Geometry: see drawing. Coordinates: mm, zero at the bounding-box minimum. A direction names the side the tool comes from. Round coordinates to 2 decimals unless told otherwise and drop trailing zeros. Order: outer loops, then holes, each group sorted by start corner. A loop starts at its lowest first (then second) coordinate and runs counter-clockwise, first axis right, second up. Notation, with made-up numbers: (39, -17) -> (80, -17) arc R20 cw to (80, -12) -> close; hole circle Ø2 at (19, -10). An arc over 180 degrees is marked (long way). One line per item, written item: value. Start each with the question number.
1) Section C-C (z = 28). Return the cut outline in (x, y) (1 decimal).
2) Section A-A (x = 4.25). Return the cut outline in (y, z), and give its area (3 significant figures).
3) Section B-B (y = 3.5). Return the cut outline in (x, z).
4) Pin query (flat end, axial travel): P1, Ø1, axis at y = 3.5, z = 32.5, coming from the +X side; P2, Ø1, axis at x = 3.5, z = 47.5, coming from the -Y side. Return the tip coordinate at first contact, or that it passes through.
5) Reachability of the marked faces 1, 2 and 3 from +Z, -Z, +X, -X, +Y, -Y: full face, straight path, thin tool, end or side. Return the list, or none.
6) Ray query, L1, parallel to Z at x = 10, y = 8.25; L2, parallel to Y at x = 5.75, z = 11.5; L3, parallel to Y at x = 6.5, z = 53 (1 decimal). Return the intervals inside material, ascending.
7) Section D-D (z = 68.5). Return the cut outline in (x, y).
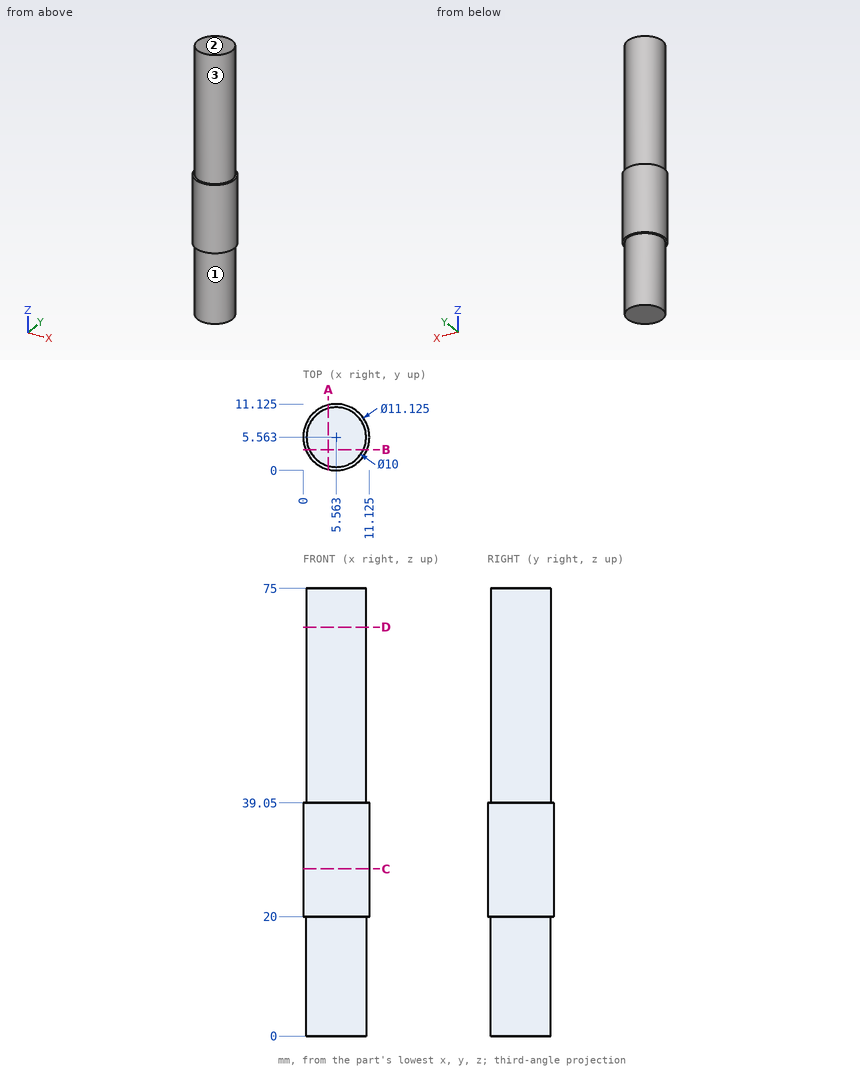
Findings:
1. outline: circle Ø11.1 at (5.6, 5.6)
2. outline: (0.16, 20) -> (0.74, 20) -> (0.74, 0) -> (10.39, 0) -> (10.39, 20) -> (10.97, 20) -> (10.97, 39.05) -> (10.39, 39.05) -> (10.39, 75) -> (0.74, 75) -> (0.74, 39.05) -> (0.16, 39.05) -> close
2. area: 746 mm2
3. outline: (0.4, 20) -> (1.01, 20) -> (1.01, 0) -> (10.12, 0) -> (10.12, 20) -> (10.73, 20) -> (10.73, 39.05) -> (10.12, 39.05) -> (10.12, 75) -> (1.01, 75) -> (1.01, 39.05) -> (0.4, 39.05) -> close
4. P1: x = 10.9
4. P2: y = 0.81
5. face 1: -Z
5. face 2: +Z, +X, -X, +Y, -Y
5. face 3: +Z
6. L1: 20 to 39.05
6. L2: 0.57 to 10.56
6. L3: 0.7 to 10.5
7. outline: circle Ø10 at (5.56, 5.56)
